For this review, take the finished solid that the model builds, in its own axes (mm). A direction names the side the tool comes from. Give positions to 0.01 mm unless a question says otherwise; leave off trailing zeros. Loops run counter-clockwise (first coordinate to the right, second up) from the corner with the lowest first, then second, coordinate; pieces in that order, holes last.
```python
from build123d import *

# Parameters (mm, degrees)
PAD035_DEPTH         = 10
SKETCH097_W          = 2
SKETCH097_H          = 7
SKETCH097_W_2        = 1.5
SKETCH097_H_2        = 6
POCKET055_DEPTH      = 10.001
POCKET055_DEPTH_BACK = 10.001
SKETCH098_R          = 2.75
POCKET056_DEPTH      = 2.001
POCKET056_DEPTH_BACK = 12.501


with BuildPart() as part:
    # Sketch096 → Pad035 (new body, symmetric)
    with BuildSketch(Plane.XY):
        Polygon((-2, 10), (11, 10), (11, 3), (12.5, 3), (12.5, -3), (11, -3), (11, -10), (-2, -10), (-2, -3), (0, -3), (0, 3), (-2, 3), align=None)
    extrude(amount=PAD035_DEPTH, both=True)

    # Sketch097 → Pocket055 (cut, two sides)
    with BuildSketch(Plane.XZ) as pocket055_sk:
        with Locations((-1, -6.5)):
            Rectangle(SKETCH097_W, SKETCH097_H)
        with Locations((-1, 6.5)):
            Rectangle(SKETCH097_W, SKETCH097_H)
        with Locations((11.75, 0)):
            Rectangle(SKETCH097_W_2, SKETCH097_H_2)
    extrude(amount=-POCKET055_DEPTH, mode=Mode.SUBTRACT)
    extrude(pocket055_sk.sketch, amount=POCKET055_DEPTH_BACK, mode=Mode.SUBTRACT)

    # Sketch098 → Pocket056 (cut, two sides)
    with BuildSketch(Plane.YZ) as pocket056_sk:
        Circle(SKETCH098_R)
    extrude(amount=-POCKET056_DEPTH, mode=Mode.SUBTRACT)
    extrude(pocket056_sk.sketch, amount=POCKET056_DEPTH_BACK, mode=Mode.SUBTRACT)


with BuildPart() as part_1:
    # Body022016 placement: moved
    add(part.part.moved(Location((137, 0, -132))))


solid = part_1.part
```
Q1. For probe 1 along Y at (x, z) = (143.25, -132); probe 2 along Z at (x, y) = (146, 0); probe 3 along X at (y, z) = (-8.25, -135.25), list the stretches that pass through material, from the lowest coordinate up.
Answers:
probe 1: y = -10 to -2.75, 2.75 to 10
probe 2: z = -142 to -134.75, -129.25 to -122
probe 3: x = 137 to 148
Q2. For pin 1 Ø1 at (x, y) = (136, 8) entering from -Z; pin 2 Ø4 at (y, z) = (2.5, -125) entering from -X; pin 3 Ø0.6 at (x, y) = (135.5, -6) entering from +Z, all flat-tipped, find the tip position at first contact; note any pin that passes through.
Answers:
pin 1: stops at z = -135
pin 2: stops at x = 137
pin 3: stops at z = -129
Q3. Consider section D-D on y = -7.25. Give the boundary of the cut face in (x, z), plus the area to 3 significant figures.
Answers:
outline: (135, -135) - (137, -135) - (137, -142) - (148, -142) - (148, -122) - (137, -122) - (137, -129) - (135, -129) - close
area: 232 mm2
Q4. Consider section B-B on z = -132. Give the boundary of the cut face in (x, y), plus the area to 4 significant figures.
Answers:
outline: (135, -10) - (148, -10) - (148, -2.75) - (137, -2.75) - (137, -3) - (135, -3) - close; (135, 3) - (137, 3) - (137, 2.75) - (148, 2.75) - (148, 10) - (135, 10) - close
area: 187.5 mm2
Q5. Mouldability with a two-part tool opening along Z and no side actions: class faces 1 (the cylindrical face through (142.423, -0.596, -134.685)), 2 (the flat face through (143, 0, -122)), 3 (the flat face through (143, 0, -142)) as +Z half, -Z half, draft (parallel to the pull), parting line (faces both ways), or undercut.
Answers:
face 1: undercut
face 2: +Z half
face 3: -Z half
Q6. Consider section A-A on y = 0. Give the boundary of the cut face in (x, z), plus the area to 4 significant figures.
Answers:
outline: (137, -142) - (149.5, -142) - (149.5, -135) - (148, -135) - (148, -134.75) - (137, -134.75) - close; (137, -129.25) - (148, -129.25) - (148, -129) - (149.5, -129) - (149.5, -122) - (137, -122) - close
area: 180.5 mm2
Q7. Machinability: for faces 4 (the flat face through (149, -3, -138)), 5 (the flat face through (149, 3, -138)), 6 (the flat face through (149, 0, -135)), 7 (the flat face through (136, -3, -132)), 8 (the flat face through (136, -6, -135)), which of the approach directions +Z, -Z, +X, -X, +Y, -Y give a long, thin tool a straight path to every point of the face, cutting with its end or side? Answer none if there is none.
Answers:
face 4: +Z, -Z, +X, -Y
face 5: +Z, -Z, +X, +Y
face 6: +X, +Y, -Y
face 7: +Z, -Z, -X
face 8: -Z, -X, +Y, -Y
Q8. Consider section C-C on x = 143.5. Give the boundary of the cut face in (y, z), plus the area to 3 significant figures.
Answers:
outline: (-10, -142) - (10, -142) - (10, -122) - (-10, -122) - close; hole circle Ø5.5 at (0, -132)
area: 376 mm2
